For this review, take the finished solid that the model builds, in its own axes (mm). A direction names the side the tool comes from. Round coordinates to 2 decimals unless told otherwise and drop trailing zeros. Loops run counter-clockwise (first coordinate to the right, second up) from the corner with the lowest first, then second, coordinate; pieces in that order, holes last. Notation, with made-up numbers: (-35.5, -13) -> (-18.5, -13) arc R13 ccw to (-18.5, 7) -> close; hole circle Ø6 at (12, 59). An arc over 180 degrees is marked (long way). One line per question, with ' | ' between items. Start each with the question number.
1. Draft analysis for pull direction X (two halves, no side actions). For faces 1 (the face through (106, 53, 0)), 2 (the face through (112.76, 0.74, 7.37)), 3 (the face through (104.8, 8.62, -4.7)), state which applies: pulls with the +X half, pulls with the -X half, needs draft (parallel to the pull), parting line crosses it, or undercut.
2. Consider section C-C (y = 0). Write out the cut boundary in (x, z), and give its area (3 significant figures).
3. Consider section A-A (x = 106). Write out the cut boundary in (y, z).
4. For pin 1 Ø8 at (y, z) = (19, 7) entering from +X; pin 2 Ø1.8 at (x, y) = (104.5, -7) entering from -Z; pin 3 Ø8 at (x, y) = (106, 0) entering from +Z; pin 4 Ø1.3 at (x, y) = (106, 7.5) entering from -Z, all flat-tipped, find the tip position at first contact; note any pin that passes through.
5. Consider section D-D (z = -4.25). Count the separate pieces of the cut face and the enclosed holes in it, and give its area (3 significant figures).
6. Wall thickness on line 1 along Y through (x, z) = (105.75, 1.25); line 2 along Y through (x, z) = (104.25, -8); line 3 along X through (y, z) = (8, -2.25): over which ranges is each line inside the solid? List them lowest first.
7. Consider section B-B (z = 5.75). Write out the cut boundary in (x, y), and give its area (3 significant figures).
8. For faces 4 (the face through (104.8, -7.3, -4.7)), 5 (the face through (110.957, -0.651, 0.367)), 6 (the face through (105, -9, -9.54)), 7 (the face through (106, 8, 0)), list the 3-axis set-ups (+Z, -Z, +X, -X, +Y, -Y) from which the entire face can be reached by the end or side of a thin tool; tool diameter is ignored.
```python
from build123d import *

# Parameters (mm, degrees)
CYLINDER004_R               = 1.35
CYLINDER004_DEPTH           = 10
CYLINDER004_PLACEMENT_ANGLE = 91
CYLINDER003_R               = 1.35
CYLINDER003_DEPTH           = 10
CYLINDER003_PITCH_ANGLE     = 90
CYLINDER002_R               = 5
CYLINDER002_DEPTH           = 20
CYLINDER002_PITCH_ANGLE     = 90
BOX_W                       = 10
BOX_H                       = 6
BOX_DEPTH                   = 22
CYLINDER001_R               = 10
CYLINDER001_DEPTH           = 106
CUT003_PITCH_ANGLE          = 90
CUT003_PLACEMENT_ANGLE      = -90


with BuildPart() as cylinder004:
    # Cylinder004 → Cylinder004 (new body)
    with BuildSketch(Plane.XY):
        Circle(CYLINDER004_R)
    extrude(amount=CYLINDER004_DEPTH)


with BuildPart() as cylinder004_1:
    # Cylinder004 placement: moved
    add(cylinder004.part.moved(Location((0, 0, 85))).rotate(Axis((0, 0, 85), (0, 1, 0)), CYLINDER004_PLACEMENT_ANGLE))


with BuildPart() as cylinder003:
    # Cylinder003 → Cylinder003 (new body)
    with BuildSketch(Plane.XY):
        Circle(CYLINDER003_R)
    extrude(amount=CYLINDER003_DEPTH)


with BuildPart() as cylinder003_1:
    # Cylinder003 pitch: moved
    add(cylinder003.part.rotate(Axis((0, 0, 0), (0, 1, 0)), CYLINDER003_PITCH_ANGLE))


with BuildPart() as cylinder003_2:
    # Cylinder003 placement: moved
    add(cylinder003_1.part.moved(Location((0, 0, 69))))


with BuildPart() as cylinder002:
    # Cylinder002 → Cylinder002 (new body)
    with BuildSketch(Plane.XY):
        Circle(CYLINDER002_R)
    extrude(amount=CYLINDER002_DEPTH)


with BuildPart() as cylinder002_1:
    # Cylinder002 pitch: moved
    add(cylinder002.part.rotate(Axis((0, 0, 0), (0, 1, 0)), CYLINDER002_PITCH_ANGLE))


with BuildPart() as cylinder002_2:
    # Cylinder002 placement: moved
    add(cylinder002_1.part.moved(Location((-10, 0, 77))))


with BuildPart() as cube:
    # Box → Box (new body)
    with BuildSketch(Plane(origin=(9.54, -3, 66), x_dir=(1, 0, 0), z_dir=(0, 0, 1))):
        with Locations((5, 3)):
            Rectangle(BOX_W, BOX_H)
    extrude(amount=BOX_DEPTH)


with BuildPart() as lever:
    # Cylinder001 → Cylinder001 (new body)
    with BuildSketch(Plane.XY.offset(24)):
        Circle(CYLINDER001_R)
    extrude(amount=CYLINDER001_DEPTH)

    # Cut: cut Cube
    add(cube.part, mode=Mode.SUBTRACT)

    # Cut001: cut Cylinder002
    add(cylinder002_2.part, mode=Mode.SUBTRACT)

    # Cut002: cut Cylinder003
    add(cylinder003_2.part, mode=Mode.SUBTRACT)

    # Cut003: cut Cylinder004
    add(cylinder004_1.part, mode=Mode.SUBTRACT)


with BuildPart() as lever_1:
    # Cut003 pitch: moved
    add(lever.part.rotate(Axis((0, 0, 0), (0, 1, 0)), CUT003_PITCH_ANGLE))


with BuildPart() as lever_2:
    # Cut003 placement: moved
    add(lever_1.part.moved(Location((106, 77, 0))).rotate(Axis((106, 77, 0), (0, 0, 1)), CUT003_PLACEMENT_ANGLE))


solid = lever_2.part
```
Answer block:
1) face 1: needs draft | face 2: parting line crosses it | face 3: undercut
2) outline: (101, -8.66) -> (101, 8.66) arc R10 ccw to start; (111, -8.66) arc R10 ccw to (111, 8.66) -> close | area: 123 mm2
3) outline: (-53, -10) -> (-11, -10) -> (-11, -9.54) -> (-9.18, -9.54) -> (-9.35, -0.02) -> (-6.65, 0.02) -> (-6.48, -9.54) -> (-5, -9.54) -> (-5, 10) -> (-53, 10) -> close; (5, -9.54) -> (6.65, -9.54) -> (6.65, 0) -> (9.35, 0) -> (9.35, -9.54) -> (11, -9.54) -> (11, -10) -> (53, -10) -> (53, 10) -> (5, 10) -> close
4) pin 1: stops at x = 115.54 | pin 2: stops at z = -9.54 | pin 3: passes through | pin 4: stops at z = 0
5) separate pieces: 1 | enclosed holes: 3 | area: 1,830 mm2
6) line 1: y = -53 to -4.99, 4.99 to 53 | line 2: y = -53 to -4.68, 4.68 to 53 | line 3: x = 96.26 to 104.65, 107.35 to 115.74
7) outline: (97.82, -53) -> (114.18, -53) -> (114.18, 53) -> (97.82, 53) -> close; hole circle Ø10 at (106, 0) | area: 1,660 mm2
8) face 4: none | face 5: +Z, -Z | face 6: -Z, +X, -X | face 7: -Z
